from build123d import *

# Parameters (mm, degrees)
SKETCH1_R           = 6
SKETCH1_R_2         = 0.6
BOSS_EXTRUDE1_DEPTH = 7.5
SKETCH1_2_R         = 0.6
BOSS_EXTRUDE2_DEPTH = 11.45


with BuildPart() as part:
    # Sketch1 → Boss-Extrude1 (new, symmetric)
    with BuildSketch(Plane.XY):
        Circle(SKETCH1_R)
        Circle(SKETCH1_R_2, mode=Mode.SUBTRACT)
    extrude(amount=BOSS_EXTRUDE1_DEPTH, both=True)

    # Sketch1<2> → Boss-Extrude2 (add, symmetric)
    with BuildSketch(Plane.XY):
        Circle(SKETCH1_2_R)
    extrude(amount=BOSS_EXTRUDE2_DEPTH, both=True)


solid = part.part
Here's how the part is built. I have some questions about the finished solid (model axes, mm). A direction names the side the tool comes from. Round coordinates to 2 decimals unless told otherwise and drop trailing zeros. Write each loop counter-clockwise with the first axis right and the second up, starting at its lowest first coordinate (ties: lowest second). Pieces come first, ordered by that corner, then holes.
1. Suppose I cut it at D-D (x = 2.5). List the corners of the cut face in (y, z) for me.
2. For faces 1 (the cylindrical face through (0.323, 0.506, -9.447)), 2 (the cylindrical face through (0.323, 0.506, 9.503)), 3 (the flat face through (0, 0, -11.45)), which set-ups out of +Z, -Z, +X, -X, +Y, -Y let a thin tool reach every point of the face, with its end or its side?
3. Suppose I cut it at A-A (y = 0). List the corners of the cut face in (x, z) for me, and give its area (3 significant figures).
4. Suppose I cut it at C-C (z = 3.25). List the corners of the cut face in (x, y) for me, and give its area (3 significant figures).
5. Will these pins go through, and if not, where does the flat tip stop? pin 1 Ø4 at (x, y) = (-3, -2) entering from -Z; pin 2 Ø2 at (x, z) = (-1, 1.5) entering from +Y; pin 3 Ø1 at (y, z) = (1, 5.5) entering from -X.
6. I need wall thicknesses on L1, parallel to Z at x = 4.75, y = 2.5; L2, parallel to Y at x = -4.25, z = 7; L3, parallel to X at y = 1.25, z = -6.25. Which ranges of each line are inside material? Lowest first, please.
Answer sheet:
1. outline: (-5.45, -7.5) - (5.45, -7.5) - (5.45, 7.5) - (-5.45, 7.5) - close
2. face 1: -Z
2. face 2: +Z
2. face 3: -Z, +X, -X, +Y, -Y
3. outline: (-6, -7.5) - (-0.6, -7.5) - (-0.6, -11.45) - (0.6, -11.45) - (0.6, -7.5) - (6, -7.5) - (6, 7.5) - (0.6, 7.5) - (0.6, 11.45) - (-0.6, 11.45) - (-0.6, 7.5) - (-6, 7.5) - close
3. area: 189 mm2
4. outline: circle Ø12 at (0, 0)
4. area: 113 mm2
5. pin 1: stops at z = -7.5
5. pin 2: stops at y = 6
5. pin 3: stops at x = -5.98
6. L1: z = -7.5 to 7.5
6. L2: y = -4.24 to 4.24
6. L3: x = -5.87 to 5.87
